For this review, take the finished solid that the model builds, in its own axes (mm). A direction names the side the tool comes from. Give positions to 0.01 mm unless a question says otherwise; leave off trailing zeros. Write each loop counter-clockwise with the first axis right and the second up, starting at its lowest first coordinate (ties: lowest second). Pieces come first, ordered by that corner, then holes.
1) Draft analysis for pull direction X (two halves, no side actions). For faces 4 (the face through (7.287, 2.028, 9.248)), 5 (the face through (44.4, 2, 5)), 6 (the face through (0, 2, 5)), state which applies: pulls with the +X half, pulls with the -X half, needs draft (parallel to the pull), parting line crosses it, or undercut.
2) We need section A-A on z = 5. Give the number of separate pieces and of enclosed holes in the cut face, and give its area (3 significant figures).
3) We need section C-C on x = 14. Give the boundary of the cut face in (y, z), and give its area (3 significant figures).
4) We need section B-B on x = 40.4. Give the boundary of the cut face in (y, z), and give its area (3 significant figures).
5) Machinability: for faces 1 (the face through (22, 1.5, 5)), 2 (the face through (37.113, 2.028, 9.248)), 3 (the face through (41.9, 2.521, 7.883)), which of the approach directions +Z, -Z, +X, -X, +Y, -Y give a long, thin tool a straight path to every point of the face, cutting with its end or side? Answer none if there is none.
6) For P1, Ø3, axis at x = 3.5, z = 6.5, coming from the +Y side; P2, Ø3, axis at x = 8, y = 5, coming from the +Z side; P3, Ø6, axis at x = 11, z = 8.5, coming from the -Y side; P4, Ø2.5, axis at x = 25, z = 5.5, coming from the -Y side, all flat-tipped, find the tip position at first contact; note any pin that passes through.
7) Wall thickness on line 1 along X through (y, z) = (0.3, 5); line 2 along Z through (x, y) = (40.4, 0.5); line 3 along X through (y, z) = (3.1, 4): over which ranges is each line inside the solid? List them lowest first.
from build123d import *

# Parameters (mm, degrees)
RESSALTO_EXTRUS_O1_DEPTH          = 10
REBAIXO_PARA_SHCS_M31_D           = 3.4
REBAIXO_PARA_SHCS_M31_CBORE_D     = 6.5
REBAIXO_PARA_SHCS_M31_CBORE_DEPTH = 3
ESBO_O4_W                         = 28.4
ESBO_O4_H                         = 5.5
CORTE_EXTRUS_O1_DEPTH             = 2.5
ESBO_O5_W                         = 28.4
ESBO_O5_H                         = 5.5
CORTE_EXTRUS_O2_DEPTH             = 2.5
FILETE1_R                         = 2.5
FILETE2_R                         = 1.5


with BuildPart() as part:
    # Esboço1 → Ressalto-extrusão1 (new body)
    with BuildSketch(Plane.XY):
        Polygon((0, 0), (12, 0), (12, 1.5), (32.4, 1.5), (32.4, 0), (44.4, 0), (44.4, 4), (36.4, 4), (36.4, 5.5), (8, 5.5), (8, 4), (0, 4), align=None)
    extrude(amount=RESSALTO_EXTRUS_O1_DEPTH)

    # Rebaixo para SHCS M31 (through all)
    with Locations(Plane(origin=(0, 4, 0), x_dir=(1, 0, 0), z_dir=(0, 1, 0))):
        with Locations((4, -5), (40.4, -5)):
            CounterBoreHole(REBAIXO_PARA_SHCS_M31_D / 2, REBAIXO_PARA_SHCS_M31_CBORE_D / 2, REBAIXO_PARA_SHCS_M31_CBORE_DEPTH)

    # Esboço4 → Corte-extrusão1 (cut)
    with BuildSketch(Plane.XY.offset(10)):
        with Locations((22.2, 2.75)):
            Rectangle(ESBO_O4_W, ESBO_O4_H)
    extrude(amount=-CORTE_EXTRUS_O1_DEPTH, mode=Mode.SUBTRACT)

    # Esboço5 → Corte-extrusão2 (cut)
    with BuildSketch(Plane(origin=(0, 0, 0), x_dir=(-1, 0, 0), z_dir=(0, 0, -1))):
        with Locations((-22.2, 2.75)):
            Rectangle(ESBO_O5_W, ESBO_O5_H)
    extrude(amount=-CORTE_EXTRUS_O2_DEPTH, mode=Mode.SUBTRACT)

    # Filete1
    filete1_edges = [part.edges().sort_by_distance(p)[0] for p in [
        (8, 2, 10),
        (0, 2, 10),
        (0, 2, 0),
        (8, 2, 0),
        (36.4, 2, 10),
        (44.4, 2, 10),
        (44.4, 2, 0),
        (36.4, 2, 0),
    ]]
    fillet(filete1_edges, radius=FILETE1_R - 0.0001)  # a hair under: the kernel refuses the full size

    # Filete2
    filete2_edges = [part.edges().sort_by_distance(p)[0] for p in [
        (36.4, 5.5, 5),
        (8, 5.5, 5),
    ]]
    fillet(filete2_edges, radius=FILETE2_R - 0.0001)  # a hair under: the kernel refuses the full size


solid = part.part
Results list:
1. face 4: undercut
1. face 5: pulls with the +X half
1. face 6: pulls with the -X half
2. separate pieces: 3
2. enclosed holes: 0
2. area: 143 mm2
3. outline: (1.5, 2.5) - (5.5, 2.5) - (5.5, 7.5) - (1.5, 7.5) - close
3. area: 20.0 mm2
4. outline: (0, 0) - (4, 0) - (4, 1.75) - (1, 1.75) - (1, 3.3) - (0, 3.3) - close; (0, 6.7) - (1, 6.7) - (1, 8.25) - (4, 8.25) - (4, 10) - (0, 10) - close
4. area: 17.1 mm2
5. face 1: +Z, -Z, -Y
5. face 2: +Z, +Y, -Y
5. face 3: +Y
6. P1: stops at y = 1
6. P2: stops at z = 9.58
6. P3: stops at y = 0
6. P4: stops at y = 1.5
7. line 1: x = 0 to 2.3, 5.7 to 12, 32.4 to 38.7, 42.1 to 44.4
7. line 2: z = 0 to 3.3, 6.7 to 10
7. line 3: x = 0 to 0.91, 7.09 to 37.31, 43.49 to 44.4
